The model under review builds one solid part; all positions refer to its coordinate system, in mm. A direction names the side the tool comes from. Give positions to 0.01 mm unless a question says otherwise; leave off trailing zeros. Write each loop counter-clockwise with the first axis right and the second up, starting at its lowest first coordinate (ties: lowest second). Pieces come first, ordered by that corner, then holes. Notation, with made-up numbers: (26.5, 8.25) - (82.5, 8.25) arc R25 cw to (82.5, 36.25) - close; hole circle Ø10 at (-39.75, 69). An arc over 180 degrees is marked (long way). Write item = value, one per line.
```python
from build123d import *

# Parameters (mm, degrees)
BOSS_EXTRUDE2_DEPTH            = 1
F_3_2_3_2_DIAMETER_HOLE1_D     = 3.2
F_3_2_3_2_DIAMETER_HOLE1_DEPTH = 1.6
F_3_2_3_2_DIAMETER_HOLE1_TIP   = 0.96137699
F_2_7_2_7_DIAMETER_HOLE1_D     = 2.7
F_2_7_2_7_DIAMETER_HOLE1_DEPTH = 1.6
F_2_7_2_7_DIAMETER_HOLE1_TIP   = 0.811161836
EDGE_FLANGE1_DEPTH             = 62
EDGE_FLANGE1_START             = 1
EDGE_FLANGE1_FLAT_DEPTH        = 1
EDGE_FLANGE1_BEND_DEPTH        = 25.5
EDGE_FLANGE1_FLAT_2_DEPTH      = 1
EDGE_FLANGE1_BEND_2_DEPTH      = 34.5
EDGE_FLANGE1_FLAT_3_DEPTH      = 1


# Sheet-metal steps are written as plain solids
with BuildPart() as part:
    # Sketch1 → Boss-Extrude2 (new body)
    with BuildSketch(Plane.XY.offset(10)):
        Polygon((-44.583280636, -10.201603144), (-24.583280636, -10.201603144), (-24.583280636, -35.201603144), (-13.583280636, -35.201603144), (-13.583280636, -31.201603144), (22.916719364, -31.201603144), (22.916719364, -22.201603144), (30.916719364, -22.201603144), (30.916719364, 39.798396856), (22.916719364, 39.798396856), (22.916719364, 52.798396856), (-17.083280636, 52.798396856), (-17.083280636, 47.798396856), (-44.583280636, 47.798396856), align=None)
    extrude(amount=BOSS_EXTRUDE2_DEPTH)

    # Ø3.2 (3.2) Diameter Hole1
    with Locations(Plane.XY.offset(11)):
        with Locations((-33.083280636, 43.798396856), (26.916719364, 26.298396856), (26.916719364, -18.701603144), (1.416719364, 49.798396856), (-19.083280636, -32.201603144)):
            Hole(F_3_2_3_2_DIAMETER_HOLE1_D / 2, depth=F_3_2_3_2_DIAMETER_HOLE1_DEPTH)
            with Locations((0, 0, -(F_3_2_3_2_DIAMETER_HOLE1_DEPTH + F_3_2_3_2_DIAMETER_HOLE1_TIP / 2))):  # 118° drill point
                Cone(0, F_3_2_3_2_DIAMETER_HOLE1_D / 2, F_3_2_3_2_DIAMETER_HOLE1_TIP, mode=Mode.SUBTRACT)

    # Ø2.7 (2.7) Diameter Hole1
    with Locations(Plane.XY.offset(11)):
        with Locations((-10.783280636, -6.994496363), (13.716719364, -6.994496363), (-10.783280636, 49.298396856), (13.716719364, 49.298396856)):
            Hole(F_2_7_2_7_DIAMETER_HOLE1_D / 2, depth=F_2_7_2_7_DIAMETER_HOLE1_DEPTH)
            with Locations((0, 0, -(F_2_7_2_7_DIAMETER_HOLE1_DEPTH + F_2_7_2_7_DIAMETER_HOLE1_TIP / 2))):  # 118° drill point
                Cone(0, F_2_7_2_7_DIAMETER_HOLE1_D / 2, F_2_7_2_7_DIAMETER_HOLE1_TIP, mode=Mode.SUBTRACT)

    # Edge-Flange1 bend section (across the edge) → Edge-Flange1 (add)
    with BuildSketch(Plane(origin=(31.916719364, 39.798396856, 10), x_dir=(-1, 0, 0), z_dir=(0, -1, 0))):
        with BuildLine():
            Line((-1, 1), (0, 1))
            ThreePointArc((0, 1), (0.292893219, 0.292893219), (1, 0))
            Line((1, 0), (1, -1))
            ThreePointArc((1, -1), (-0.414213562, -0.414213562), (-1, 1))
        make_face()
    extrude(amount=EDGE_FLANGE1_DEPTH)

    # Edge-Flange1 profile (on flange) → Edge-Flange1 flat (add)
    with BuildSketch(Plane(origin=(31.916719364, 0, 10), x_dir=(0, -1, 0), z_dir=(1, 0, 0)).offset(EDGE_FLANGE1_START)):
        Polygon((-39.798396856, 1), (22.201603144, 1), (22.201603144, 19), (6.871603144, 19), (6.871603144, 23), (4.871603144, 23), (4.871603144, 19), (-16.468396856, 19), (-16.468396856, 23), (-18.468396856, 23), (-18.468396856, 19), (-39.798396856, 19), align=None)
    extrude(amount=-EDGE_FLANGE1_FLAT_DEPTH)

    # Edge-Flange1 bend section 2 (across the edge) → Edge-Flange1 bend (add)
    with BuildSketch(Plane(origin=(-44.583280636, 48.798396856, 10), x_dir=(0, -1, 0), z_dir=(1, 0, 0))):
        with BuildLine():
            Line((-1, 1), (0, 1))
            ThreePointArc((0, 1), (0.292893219, 0.292893219), (1, 0))
            Line((1, 0), (1, -1))
            ThreePointArc((1, -1), (-0.414213562, -0.414213562), (-1, 1))
        make_face()
    extrude(amount=EDGE_FLANGE1_BEND_DEPTH)

    # Edge-Flange1 profile 2 (on flange) → Edge-Flange1 flat 2 (add)
    with BuildSketch(Plane(origin=(0, 48.798396856, 10), x_dir=(1, 0, 0), z_dir=(0, 1, 0)).offset(EDGE_FLANGE1_START)):
        Polygon((-19.083280636, 1), (-19.083280636, 19), (-30.833280636, 19), (-30.833280636, 23), (-32.833280636, 23), (-32.833280636, 19), (-44.583280636, 19), (-44.583280636, 1), align=None)
    extrude(amount=-EDGE_FLANGE1_FLAT_2_DEPTH)

    # Edge-Flange1 bend section 3 (across the edge) → Edge-Flange1 bend 2 (add)
    with BuildSketch(Plane(origin=(22.916719364, -32.201603144, 10), x_dir=(0, 1, 0), z_dir=(-1, 0, 0))):
        with BuildLine():
            Line((-1, 1), (0, 1))
            ThreePointArc((0, 1), (0.292893219, 0.292893219), (1, 0))
            Line((1, 0), (1, -1))
            ThreePointArc((1, -1), (-0.414213562, -0.414213562), (-1, 1))
        make_face()
    extrude(amount=EDGE_FLANGE1_BEND_2_DEPTH)

    # Edge-Flange1 profile 3 (on flange) → Edge-Flange1 flat 3 (add)
    with BuildSketch(Plane(origin=(0, -32.201603144, 10), x_dir=(-1, 0, 0), z_dir=(0, -1, 0)).offset(EDGE_FLANGE1_START)):
        Polygon((11.583280636, 1), (11.583280636, 19), (-4.666719364, 19), (-4.666719364, 23), (-6.666719364, 23), (-6.666719364, 19), (-22.916719364, 19), (-22.916719364, 1), align=None)
    extrude(amount=-EDGE_FLANGE1_FLAT_3_DEPTH)


solid = part.part
```
1. Take a section at D-D on x = -8. Give the boundary of the cut face in (y, z), and give its area (3 significant figures).
Findings below:
outline = (-33.2, -9) - (-32.2, -9) - (-32.2, 9) arc R1 cw to (-31.2, 10) - (52.8, 10) - (52.8, 11) - (-31.2, 11) arc R2 ccw to (-33.2, 9) - close
area = 104 mm²
2. Draft analysis for pull direction X (two halves, no side actions). For faces 4 (the flat face through (-44.583, 33.3, 10.6)), 5 (the cylindrical face through (28.096, 27.38, 10.493)), 6 (the flat face through (6, -33.202, 0)), state which applies: +X half, -X half, draft (parallel to the pull), parting line (faces both ways), or undercut.
Findings below:
face_4 = -X half
face_5 = undercut
face_6 = draft
3. Take a section at C-C on y = -13. Give the boundary of the cut face in (x, z).
Findings below:
outline = (-24.58, 10) - (30.92, 10) arc R1 cw to (31.92, 9) - (31.92, -9) - (32.92, -9) - (32.92, 9) arc R2 ccw to (30.92, 11) - (-24.58, 11) - close
4. Take a section at A-A on z = 3.75. Give the boundary of the cut face in (x, y), and give its area (3 significant figures).
Findings below:
outline = (-44.58, 48.8) - (-19.08, 48.8) - (-19.08, 49.8) - (-44.58, 49.8) - close; (-11.58, -33.2) - (22.92, -33.2) - (22.92, -32.2) - (-11.58, -32.2) - close; (31.92, -22.2) - (32.92, -22.2) - (32.92, 39.8) - (31.92, 39.8) - close
area = 122 mm²
5. Insertion check: P1, Ø1.6, axis at y = -32, z = -1.5, coming from the -X side; P2, Ø1.1, axis at x = 32.5, y = 24, coming from the -Z side; P3, Ø11, axis at x = -30, z = 1, coming from the +Y side; P4, Ø1.9, axis at x = 1.42, y = 49.8, coming from the -Z side. Each pin has a flat end and moves straight along its axis. Give the tip position at first contact, or say it passes through.
Findings below:
P1 = -11.58
P2 = -9
P3 = 49.8
P4 = through
6. For line 1 (X direction, y = -11.5, z = 5); line 2 (Y direction, x = -30.5, z = 5.5); line 3 (Z direction, x = 28.5, y = -22), list the stretches that pass through material, from the lowest coordinate up. Write a range as from..to.
Findings below:
line_1 = 31.92..32.92
line_2 = 48.8..49.8
line_3 = 10..11
7. Machinability: for faces 1 (the flat face through (32.4, -22.202, 3.3)), 2 (the flat face through (-19.083, 49, 1)), 3 (the flat face through (32.4, 39.798, 3.2)), which of the approach directions +Z, -Z, +X, -X, +Y, -Y give a long, thin tool a straight path to every point of the face, cutting with its end or side? Answer none if there is none.
Findings below:
face_1 = +Z, -Z, +X, -Y
face_2 = +Z, -Z, +Y
face_3 = +Z, -Z, +X, +Y
8. Take a section at B-B on x = 13.5. Give the boundary of the cut face in (y, z).
Findings below:
outline = (-33.2, -9) - (-32.2, -9) - (-32.2, 9) arc R1 cw to (-31.2, 10) - (-8.33, 10) - (-8.33, 11) - (-31.2, 11) arc R2 ccw to (-33.2, 9) - close; (-5.66, 10) - (47.97, 10) - (47.97, 11) - (-5.66, 11) - close; (50.63, 10) - (52.8, 10) - (52.8, 11) - (50.63, 11) - close
